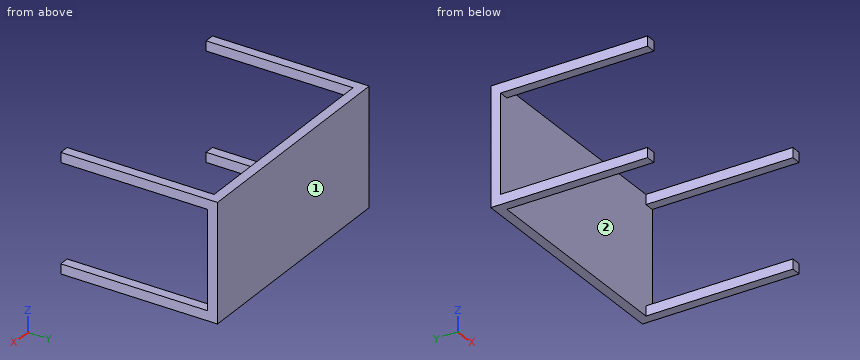
```python
from build123d import *

# Parameters (mm, degrees)
SKETCH1_W           = 1828.8
SKETCH1_H           = 609.6
BOSS_EXTRUDE1_DEPTH = 50.8
SKETCH2_W           = 50.8
SKETCH2_H           = 50.8
BOSS_EXTRUDE2_DEPTH = 762
SKETCH3_W           = 609.6
SKETCH3_H           = 812.8
CUT_EXTRUDE1_DEPTH  = 1338.304572639
SKETCH4_W           = 50.8
SKETCH4_H           = 50.8
BOSS_EXTRUDE3_DEPTH = 762


with BuildPart() as part:
    # Sketch1 → Boss-Extrude1 (new body)
    with BuildSketch(Plane(origin=(0, 0, 0), x_dir=(1, 0, 0), z_dir=(0, 1, 0))):
        Rectangle(SKETCH1_W, SKETCH1_H)
    extrude(amount=BOSS_EXTRUDE1_DEPTH)

    # Sketch2 → Boss-Extrude2 (add)
    with BuildSketch(Plane.XZ):
        with Locations((-889, 279.4)):
            Rectangle(SKETCH2_W, SKETCH2_H)
        with Locations((-889, -279.4)):
            Rectangle(SKETCH2_W, SKETCH2_H)
        with Locations((889, 279.4)):
            Rectangle(SKETCH2_W, SKETCH2_H)
        with Locations((889, -279.4)):
            Rectangle(SKETCH2_W, SKETCH2_H)
    extrude(amount=BOSS_EXTRUDE2_DEPTH)

    # Sketch3 → Cut-Extrude1 (cut, through all)
    with BuildSketch(Plane.XY.offset(304.8)):
        with Locations((609.6, -355.6)):
            Rectangle(SKETCH3_W, SKETCH3_H)
    extrude(amount=-CUT_EXTRUDE1_DEPTH, mode=Mode.SUBTRACT)

    # Sketch4 → Boss-Extrude3 (add)
    with BuildSketch(Plane.XZ):
        with Locations((279.4, 279.4)):
            Rectangle(SKETCH4_W, SKETCH4_H)
        with Locations((279.4, -279.4)):
            Rectangle(SKETCH4_W, SKETCH4_H)
    extrude(amount=BOSS_EXTRUDE3_DEPTH)


solid = part.part
```
The model under review builds one solid part; all positions refer to its coordinate system, in mm. Face numbers are marked on the shaded views. Round coordinates to 2 decimals unless told otherwise and drop trailing zeros. Order: outer loops, then holes, each group sorted by start corner. A loop starts at its lowest first (then second) coordinate and runs counter-clockwise, first axis right, second up.
Item 1: For pin 1 (6 mm diameter, centred on x = -28.5, z = 207, fed in from -Y), flat-tipped, find the tip position at first contact; note if it passes through.
Working result:
pin 1: stops at y = 0
Item 2: Add section B-B, the plane z = 31.5. State the section outline as (x, y) points.
Working result:
outline: (-914.4, 0) - (304.8, 0) - (304.8, 50.8) - (-914.4, 50.8) - close
Item 3: To check wall thickness, follow probe 1 along X at (y, z) = (-144, 261.5); probe 2 along Y at (x, z) = (-506.5, -5.5). State the ranges of each line that lie inside material, in increasing order.
Working result:
probe 1: x = -914.4 to -863.6, 254 to 304.8
probe 2: y = 0 to 50.8
Item 4: Draft analysis for pull direction X (two halves, no side actions). For the marked faces 1 and 2, state which applies: released by +X, released by -X, zero draft, split by the parting line, or undercut.
Working result:
face 1: zero draft
face 2: undercut
Item 5: Add section A-A, the plane y = -62. State the section outline as (x, z) points.
Working result:
outline: (-914.4, -304.8) - (-863.6, -304.8) - (-863.6, -254) - (-914.4, -254) - close; (-914.4, 254) - (-863.6, 254) - (-863.6, 304.8) - (-914.4, 304.8) - close; (254, -304.8) - (304.8, -304.8) - (304.8, -254) - (254, -254) - close; (254, 254) - (304.8, 254) - (304.8, 304.8) - (254, 304.8) - close
Item 6: Add section C-C, the plane x = -614. State the section outline as (y, z) points, and give its area (3 significant figures).
Working result:
outline: (0, -304.8) - (50.8, -304.8) - (50.8, 304.8) - (0, 304.8) - close
area: 31,000 mm2
